Can you work these out from the model? Positions are in its coordinate system, mm. A direction names the side the tool comes from. Give positions to 0.01 mm unless a question says otherwise; leave off trailing zeros. Order: outer loops, then holes, each group sorted by start corner. A loop starts at its lowest first (then second) coordinate and runs counter-clockwise, first axis right, second up. Notation, with made-up numbers: (-5.75, 60) - (-1.75, 60) arc R24 cw to (-1.75, 88) - close; hole circle Ø3 at (-5, 75.25). An arc over 180 degrees is marked (long way). Answer as CSV lines item,"result".
```python
from build123d import *

# Parameters (mm, degrees)
F0_W        = 127
F0_H        = 76.2
F1_DEPTH    = 12.7
F2_R        = 6.35
F3_DEPTH    = 12.701
F4_W        = 19.05
F4_H        = 38.1
F6_W        = 6.35
F6_H        = 10.16
F8_R        = 5.08
F9_S7_R     = 17.0504603439
F9_T8_DEPTH = 29
F10_SIZE    = 5.08


# Not quite as in the source:
# - a fillet or chamfer that OpenCascade refuses, or shapes differently, is made with other operations: its cross-section is extruded or revolved along the edge and cut away or added


with BuildPart() as f1:
    # F0 (on Top) → F1 (new body)
    with BuildSketch(Plane.XY):
        Rectangle(F0_W, F0_H)
    extrude(amount=F1_DEPTH)

    # F2 (on face) → F3 (cut, through all)
    with BuildSketch(Plane.XY.offset(12.7)):
        with Locations((50.8, -25.4)):
            Circle(F2_R)
        with Locations((50.8, 25.4)):
            Circle(F2_R)
        with Locations((-50.8, 25.4)):
            Circle(F2_R)
        with Locations((-50.8, -25.4)):
            Circle(F2_R)
    extrude(amount=-F3_DEPTH, mode=Mode.SUBTRACT)

    # F4 (on Front) → F5 (revolve)
    with BuildSketch(Plane.XZ):
        with Locations((9.525, 31.75)):
            Rectangle(F4_W, F4_H)
    revolve(axis=Axis((0, 0, 31.75), (0, 0, 1)))

    # F6 (on Front) → F7 (revolve, cut)
    with BuildSketch(Plane.XZ):
        with Locations((20.2254603439, 35.56)):
            Rectangle(F6_W, F6_H)
    revolve(axis=Axis((0, 0, 50.8), (0, 0, 1)), mode=Mode.SUBTRACT)

    # F8
    f8_edges = [f1.edges().sort_by_distance(p)[0] for p in [
        (-19.05, 0, 50.8),
    ]]
    fillet(f8_edges, radius=F8_R)

    # F9: chamfer of 5.08 on 3 edges, made by hand

    # F9_s1 → F9_t2 (revolve)
    with BuildSketch(Plane.XZ):
        Polygon((19.05, 17.78), (24.13, 12.7), (19.05, 12.7), align=None)
    revolve(axis=Axis((0, 0, 12.7), (0, 0, 1)))


with BuildPart() as f9_tool4:
    # F9_s5 → F9_t6 (revolve)
    with BuildSketch(Plane.XZ):
        Polygon((13.97, 30.48), (19.05, 25.4), (19.05, 30.48), align=None)
    revolve(axis=Axis((0, 0, 30.48), (0, 0, 1)))

    # F9_s7 → F9_t8 (cut, symmetric)
    with BuildSketch(Plane.XY.offset(27.9)):
        Circle(F9_S7_R)
    extrude(amount=F9_T8_DEPTH, both=True, mode=Mode.SUBTRACT)


with BuildPart() as f1_1:
    add(f1.part)

    # F9_t3: cut F9_tool4
    add(f9_tool4.part, mode=Mode.SUBTRACT)

    # F10
    f10_edges = [f1_1.edges().sort_by_distance(p)[0] for p in [
        (0, -38.1, 12.7),
        (63.5, 0, 12.7),
        (0, 38.1, 12.7),
        (-63.5, 0, 12.7),
    ]]
    chamfer(f10_edges, length=F10_SIZE)


solid = f1_1.part
```
1) I need wall thicknesses on line 1 along Y through (x, z) = (50.8, 3); line 2 along Y through (x, z) = (-50.8, 9.25); line 3 along X through (y, z) = (-25, 9). Which ranges of each line are inside material? Lowest first, please. Write a range as [from, to].
Answer block:
line 1,"[-38.1, -31.75], [-19.05, 19.05], [31.75, 38.1]"
line 2,"[-36.47, -31.75], [-19.05, 19.05], [31.75, 36.47]"
line 3,"[-62.12, -57.14], [-44.46, 44.46], [57.14, 62.12]"
2) I want a section at C-C on y = 0. Write out the boundary of the cut face in (x, z), plus the area to 3 significant figures.
Answer block:
outline,"(-63.5, 0) - (63.5, 0) - (63.5, 7.62) - (58.42, 12.7) - (24.13, 12.7) - (19.05, 17.78) - (19.05, 25.4) - (17.05, 27.4) - (17.05, 40.64) - (19.05, 40.64) - (19.05, 45.72) arc R5.08 ccw to (13.97, 50.8) - (-13.97, 50.8) arc R5.08 ccw to (-19.05, 45.72) - (-19.05, 40.64) - (-17.05, 40.64) - (-17.05, 27.4) - (-19.05, 25.4) - (-19.05, 17.78) - (-24.13, 12.7) - (-58.42, 12.7) - (-63.5, 7.62) - close"
area,"3,000 mm2"
3) I want a section at A-A on x = 50.8. Write out the boundary of the cut face in (y, z), plus the area to 3 significant figures.
Answer block:
outline,"(-38.1, 0) - (-31.75, 0) - (-31.75, 12.7) - (-33.02, 12.7) - (-38.1, 7.62) - close; (-19.05, 0) - (19.05, 0) - (19.05, 12.7) - (-19.05, 12.7) - close; (31.75, 0) - (38.1, 0) - (38.1, 7.62) - (33.02, 12.7) - (31.75, 12.7) - close"
area,"619 mm2"
4) I want a section at B-B on y = -25.4. Write out the boundary of the cut face in (x, z).
Answer block:
outline,"(-63.5, 0) - (-57.15, 0) - (-57.15, 12.7) - (-58.42, 12.7) - (-63.5, 7.62) - close; (-44.45, 0) - (44.45, 0) - (44.45, 12.7) - (-44.45, 12.7) - close; (57.15, 0) - (63.5, 0) - (63.5, 7.62) - (58.42, 12.7) - (57.15, 12.7) - close"
5) Which directions (+Z, -Z, +X, -X, +Y, -Y) give clear straight access to the entire face, cutting with the end or side of a thin tool? Please do faces 4 (the cylindrical face through (56.666, 22.968, 6.439)), 5 (the flat face through (14, -10, 40.64)).
Answer block:
face 4,"+Z, -Z"
face 5,"none"
6) If we mould it in two halves opening along Z, with no side actions, what happens to faces 1 (the cylindrical face through (-15.12, -11.59, 43.22)), 2 (the conical face through (-2.521, 19.203, 17.462)), 3 (the cylindrical face through (16.263, 5.121, 34.112))? For each: +Z half, -Z half, draft (parallel to the pull), parting line (faces both ways), or undercut.
Answer block:
face 1,"draft"
face 2,"+Z half"
face 3,"undercut"
7) I want a section at D-D on z = 16.5. Write out the boundary of the cut face in (x, y).
Answer block:
outline,"circle Ø40.66 at (0, 0)"
8) I'm going to push flat-ended pins straight in: P1, Ø20.5, axis at x = -50.8, y = 25.4, coming from the +Z side; P2, Ø6, axis at y = -17.5, z = 34.5, coming from the -X side; P3, Ø6, axis at y = 28, z = 11.5, coming from the -X side. Where does each tip first touch, or does it pass through?
Answer block:
P1,"z = 12.7"
P2,"x = -8.97"
P3,"x = -62.62"
